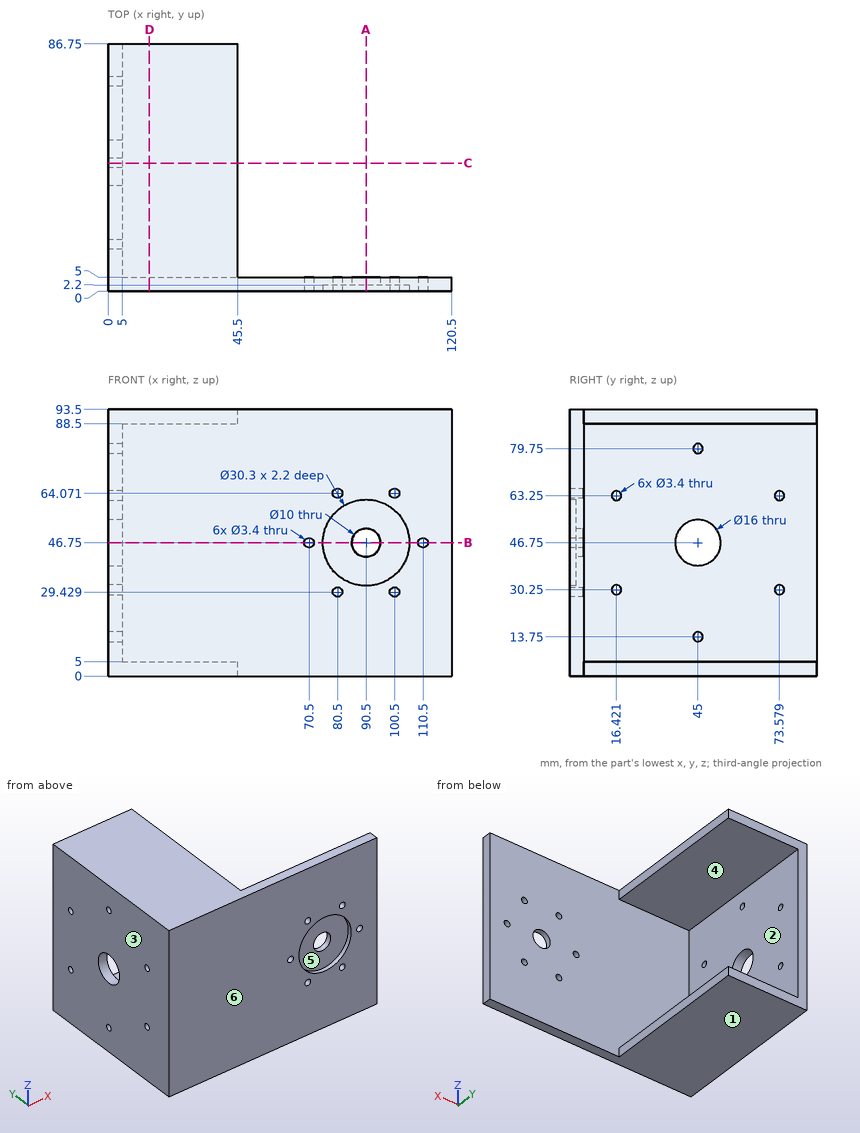
Part print with two shaded views. Sizes in mm from the minimum x, y, z corner. A direction names the side the tool comes from. Coordinates: 2 decimals unless noted, no trailing zeros. Loops run counter-clockwise (first coordinate to the right, second up) from the corner with the lowest first, then second, coordinate; pieces in that order, holes last. Notation, with made-up numbers: M 43.25,-37.5 L 102.25,-37.5 A15 ccw 102.25,-28.5 Z; hole C 0,37.5 d8. An arc over 180 degrees is marked long. Use CSV: the item, a comma, the result in double quotes. Start each with the question number.
1. Tool access for the marked faces 4, 5 and 6: list every direction of +Z, -Z, +X, -X, +Y, -Y with a clear straight run to the whole face (end or side of a thin tool).
2. Band-saw the part on C-C, the plane y = 45. List the corners of the cut face in (x, z).
3. Band-saw the part on A-A, the plane x = 90.5. List the corners of the cut face in (y, z), then the cut area to 3 significant figures.
4. Band-saw the part on D-D, the plane x = 14.5. List the corners of the cut face in (y, z).
5. Probe probe 1 along Y at (x, z) = (1.75, 30.25); probe 2 along Z at (x, y) = (27.5, 81); probe 3 along X at (y, z) = (3.75, 46.75). List the from-to ranges inside material, lowest first. Write a range as [from, to].
6. Two-plate mould, pull along Z, no slides. Class the marked faces 1, 2 and 3: pulls with the +Z half, pulls with the -Z half, needs draft (parallel to the pull), parting line crosses it, or undercut.
7. Flat gauge pins, fed straight in: pin 1 (4 mm diameter, centred on y = 19.5, z = 38, fed in from -X); pin 2 (1 mm diameter, centred on y = 64, z = 41.5, fed in from +X); pin 3 (2.5 mm diameter, centred on y = 45, z = 3, fed in from +X); pin 4 (5.5 mm diameter, centred on x = 100.5, z = 29.43, fed in from +Y). Where does each tip first touch, or does it go through?
8. Band-saw the part on B-B, the plane z = 46.75. List the corners of the cut face in (x, y).
Entries:
1,face 4,"+X, +Y"
1,face 5,"-Y"
1,face 6,"+Z, -Z, +X, -X, -Y"
2,outline,"M 0,0 L 45.5,0 L 45.5,5 L 5,5 L 5,12.05 L 0,12.05 Z; M 0,15.45 L 5,15.45 L 5,38.75 L 0,38.75 Z; M 0,54.75 L 5,54.75 L 5,78.05 L 0,78.05 Z; M 0,81.45 L 5,81.45 L 5,88.5 L 45.5,88.5 L 45.5,93.5 L 0,93.5 Z"
3,outline,"M 0,0 L 5,0 L 5,41.75 L 2.2,41.75 L 2.2,31.6 L 0,31.6 Z; M 0,61.9 L 2.2,61.9 L 2.2,51.75 L 5,51.75 L 5,93.5 L 0,93.5 Z"
3,area,"373 mm2"
4,outline,"M 0,0 L 86.75,0 L 86.75,5 L 5,5 L 5,88.5 L 86.75,88.5 L 86.75,93.5 L 0,93.5 Z"
5,probe 1,"y = [0, 14.72], [18.12, 71.88], [75.28, 86.75]"
5,probe 2,"z = [0, 5], [88.5, 93.5]"
5,probe 3,"x = [0, 68.8], [72.2, 85.5], [95.5, 108.8], [112.2, 120.5]"
6,face 1,"pulls with the -Z half"
6,face 2,"undercut"
6,face 3,"needs draft"
7,pin 1,"stops at x = 0"
7,pin 2,"stops at x = 5"
7,pin 3,"stops at x = 45.5"
7,pin 4,"stops at y = 5"
8,outline,"M 0,0 L 68.8,0 L 68.8,5 L 5,5 L 5,37 L 0,37 Z; M 0,53 L 5,53 L 5,86.75 L 0,86.75 Z; M 72.2,0 L 75.35,0 L 75.35,2.2 L 85.5,2.2 L 85.5,5 L 72.2,5 Z; M 95.5,2.2 L 105.65,2.2 L 105.65,0 L 108.8,0 L 108.8,5 L 95.5,5 Z; M 112.2,0 L 120.5,0 L 120.5,5 L 112.2,5 Z"
